from build123d import *

# Parameters (mm, degrees)
ESTRUSIONE_ESTRUSIONE1_DEPTH = 100


with BuildPart() as part:
    # Schizzo1 → Estrusione-Estrusione1 (new body)
    with BuildSketch(Plane.XY):
        with BuildLine():
            Line((-30.15, 14), (-32.65, 14))
            Line((-32.65, 14), (-32.65, 8.9))
            Line((-32.65, 8.9), (-30.45, 8.9))
            Line((-30.45, 8.9), (-30.45, 7.8))
            Line((-30.45, 7.8), (-20.55, 7.8))
            Line((-20.55, 7.8), (-20.55, 0))
            Line((-20.55, 0), (-30.45, 0))
            Line((-30.45, 0), (-30.45, -2.2))
            Line((-30.45, -2.2), (-32.65, -2.2))
            Line((-32.65, -2.2), (-32.65, -5.3))
            Line((-32.65, -5.3), (-31.15, -5.3))
            Line((-31.15, -5.3), (-31.15, -3.3))
            Line((-31.15, -3.3), (-28.75, -3.3))
            Line((-28.75, -3.3), (-28.75, -5.3))
            Line((-28.75, -5.3), (-25.45, -5.3))
            Line((-25.45, -5.3), (-25.45, -3.8))
            Line((-25.45, -3.8), (-27.25, -3.8))
            Line((-27.25, -3.8), (-27.25, -1.8))
            Line((-27.25, -1.8), (-22.05, -1.8))
            Line((-22.05, -1.8), (-22.05, -5.3))
            Line((-22.05, -5.3), (-18.85, -5.3))
            Line((-18.85, -5.3), (-18.85, 7.8))
            Line((-18.85, 7.8), (-15.821542758, 7.8))
            ThreePointArc((-15.821542758, 7.8), (-16.273540604, 4.846345824), (-14.423395659, 2.5))
            Line((-14.423395659, 2.5), (-14.074102014, 2.5))
            Line((-14.074102014, 2.5), (-14.074102014, 4.405182935))
            ThreePointArc((-14.074102014, 4.405182935), (-12.647585955, 7.8), (-11.221069895, 4.405182935))
            Line((-11.221069895, 4.405182935), (-11.221069895, 2.5))
            Line((-11.221069895, 2.5), (-10.87177625, 2.5))
            ThreePointArc((-10.87177625, 2.5), (-9.021631305, 4.846345824), (-9.473629151, 7.8))
            Line((-9.473629151, 7.8), (0, 7.8))
            Line((0, 7.8), (0, 9.4))
            Line((0, 9.4), (-29.15, 9.4))
            Line((-29.15, 9.4), (-29.15, 10.5))
            Line((-29.15, 10.5), (-30.15, 10.5))
            Line((-30.15, 10.5), (-30.15, 14))
        make_face()
        with BuildLine():
            Line((29.15, 9.4), (0, 9.4))
            Line((0, 9.4), (0, 7.8))
            Line((0, 7.8), (9.473629151, 7.8))
            ThreePointArc((9.473629151, 7.8), (9.021631305, 4.846345824), (10.87177625, 2.5))
            Line((10.87177625, 2.5), (11.221069895, 2.5))
            Line((11.221069895, 2.5), (11.221069895, 4.405182935))
            ThreePointArc((11.221069895, 4.405182935), (12.647585955, 7.8), (14.074102014, 4.405182935))
            Line((14.074102014, 4.405182935), (14.074102014, 2.5))
            Line((14.074102014, 2.5), (14.423395659, 2.5))
            ThreePointArc((14.423395659, 2.5), (16.273540604, 4.846345824), (15.821542758, 7.8))
            Line((15.821542758, 7.8), (18.85, 7.8))
            Line((18.85, 7.8), (18.85, -5.3))
            Line((18.85, -5.3), (22.05, -5.3))
            Line((22.05, -5.3), (22.05, -1.8))
            Line((22.05, -1.8), (27.25, -1.8))
            Line((27.25, -1.8), (27.25, -3.8))
            Line((27.25, -3.8), (25.45, -3.8))
            Line((25.45, -3.8), (25.45, -5.3))
            Line((25.45, -5.3), (28.75, -5.3))
            Line((28.75, -5.3), (28.75, -3.3))
            Line((28.75, -3.3), (31.15, -3.3))
            Line((31.15, -3.3), (31.15, -5.3))
            Line((31.15, -5.3), (32.65, -5.3))
            Line((32.65, -5.3), (32.65, -2.2))
            Line((32.65, -2.2), (30.45, -2.2))
            Line((30.45, -2.2), (30.45, 0))
            Line((30.45, 0), (20.55, 0))
            Line((20.55, 0), (20.55, 7.8))
            Line((20.55, 7.8), (30.45, 7.8))
            Line((30.45, 7.8), (30.45, 8.9))
            Line((30.45, 8.9), (32.65, 8.9))
            Line((32.65, 8.9), (32.65, 14))
            Line((32.65, 14), (30.15, 14))
            Line((30.15, 14), (30.15, 10.5))
            Line((30.15, 10.5), (29.15, 10.5))
            Line((29.15, 10.5), (29.15, 9.4))
        make_face()
    extrude(amount=ESTRUSIONE_ESTRUSIONE1_DEPTH)


solid = part.part
The model under review builds one solid part; all positions refer to its coordinate system, in mm. A direction names the side the tool comes from. Coordinates: 2 decimals unless noted, no trailing zeros. Write each loop counter-clockwise with the first axis right and the second up, starting at its lowest first coordinate (ties: lowest second). Pieces come first, ordered by that corner, then holes. Notation, with made-up numbers: M 46,-13.5 L 60,-13.5 A17 cw 60,18.5 Z; hole C 81.5,68 d1. An arc over 180 degrees is marked long. Put each result on its own line as item: value.
1) Add section C-C on x = 4.5. Give the boundary of the cut face in (y, z).
Computed:
outline: M 7.8,0 L 9.4,0 L 9.4,100 L 7.8,100 Z
2) Clearance check with flat-ended pins moving along their axes: pin 1 Ø1.5 at (x, y) = (-17, -0.5) entering from +Z; pin 2 Ø4 at (y, z) = (2.5, 43.5) entering from -X; pin 3 Ø1 at (y, z) = (6.5, 40) entering from +X; pin 4 Ø0.8 at (x, z) = (-29.5, 42.5) entering from +Y. State where each tip first meets the part, or that it passes through.
Computed:
pin 1: passes through
pin 2: stops at x = -20.55
pin 3: stops at x = 20.55
pin 4: stops at y = 10.5
3) Add section B-B on y = 6. Give the boundary of the cut face in (x, z), then the cut area to 3 significant figures.
Computed:
outline: M -20.55,0 L -18.85,0 L -18.85,100 L -20.55,100 Z; M -16.39,0 L -14.63,0 L -14.63,100 L -16.39,100 Z; M -10.66,0 L -8.9,0 L -8.9,100 L -10.66,100 Z; M 8.9,0 L 10.66,0 L 10.66,100 L 8.9,100 Z; M 14.63,0 L 16.39,0 L 16.39,100 L 14.63,100 Z; M 18.85,0 L 20.55,0 L 20.55,100 L 18.85,100 Z
area: 1,040 mm2
4) Add section A-A on y = 1.5. Give the boundary of the cut face in (x, z), then the cut area to 3 significant figures.
Computed:
outline: M -20.55,0 L -18.85,0 L -18.85,100 L -20.55,100 Z; M 18.85,0 L 20.55,0 L 20.55,100 L 18.85,100 Z
area: 340 mm2
5) Draft analysis for pull direction Y (two halves, no side actions). For faces 4 (the flat face through (-32, -2.2, 49)), 5 (the flat face through (-3, 8, 100)), 6 (the flat face through (-30, -3.3, 49)), state which applies: released by +Y, released by -Y, zero draft, split by the parting line, or undercut.
Computed:
face 4: undercut
face 5: zero draft
face 6: released by -Y
6) For faces 1 (the flat face through (-18.85, 1, 49)), 2 (the flat face through (-20.55, 4, 49)), 3 (the flat face through (-27.25, -3, 49)), list the 3-axis set-ups (+Z, -Z, +X, -X, +Y, -Y) from which the entire face can be reached by the end or side of a thin tool; tool diameter is ignored.
Computed:
face 1: +Z, -Z, -Y
face 2: +Z, -Z, -X
face 3: +Z, -Z
7) Wall thickness on probe 1 along X at (y, z) = (5.5, 87); probe 2 along X at (y, z) = (-2.5, 14); probe 3 along X at (y, z) = (-4.5, 77): over which ranges is each line inside the solid? List them lowest first. Write a range as [from, to].
Computed:
probe 1: x = [-20.55, -18.85], [-16.39, -14.62], [-10.67, -8.91], [8.91, 10.67], [14.62, 16.39], [18.85, 20.55]
probe 2: x = [-32.65, -27.25], [-22.05, -18.85], [18.85, 22.05], [27.25, 32.65]
probe 3: x = [-32.65, -31.15], [-28.75, -25.45], [-22.05, -18.85], [18.85, 22.05], [25.45, 28.75], [31.15, 32.65]
